from build123d import *

# Parameters (mm, degrees)
SKETCH_1_W      = 44.72
SKETCH_1_H      = 61.65
EXTRUDE_1_DEPTH = 1.125
FILLET_1_R      = 1
SKETCH_2_W      = 37.22
SKETCH_2_H      = 49.65
EXTRUDE_2_DEPTH = 0.78


with BuildPart() as part:
    # 草图1 → 凸台-拉伸1 (new body)
    with BuildSketch(Plane(origin=(0, 0, 0), x_dir=(1, 0, 0), z_dir=(0, 1, 0))):
        with Locations((-1.696923077, -14.271057692)):
            Rectangle(SKETCH_1_W, SKETCH_1_H)
    extrude(amount=EXTRUDE_1_DEPTH)

    # 圆角1
    fillet_1_edges = [part.edges().sort_by_distance(p)[0] for p in [
        (-24.056923077, 0.5625, -16.553942308),
        (20.663076923, 0.5625, -16.553942308),
        (20.663076923, 0.5625, 45.096057692),
        (-24.056923077, 0.5625, 45.096057692),
    ]]
    fillet(fillet_1_edges, radius=FILLET_1_R)

    # 草图2 → 凸台-拉伸2 (add)
    with BuildSketch(Plane.XZ):
        with Locations((-1.696923077, 14.731057692)):
            Rectangle(SKETCH_2_W, SKETCH_2_H)
    extrude(amount=EXTRUDE_2_DEPTH)


solid = part.part
Here's how the part is built. I have some questions about the finished solid (model axes, mm). Coordinates: 2 decimals unless noted, no trailing zeros. Order: outer loops, then holes, each group sorted by start corner. A loop starts at its lowest first (then second) coordinate and runs counter-clockwise, first axis right, second up.
Item 1: If we section it at B-B on x = -5: List the corners of the cut face in (y, z) for me (3 decimals).
Result sheet:
outline: (-0.78, -10.094) - (0, -10.094) - (0, -16.554) - (1.125, -16.554) - (1.125, 45.096) - (0, 45.096) - (0, 39.556) - (-0.78, 39.556) - close
Item 2: If we section it at A-A on z = 25.5: List the corners of the cut face in (x, y) for me (3 decimals).
Result sheet:
outline: (-24.057, 0) - (-20.307, 0) - (-20.307, -0.78) - (16.913, -0.78) - (16.913, 0) - (20.663, 0) - (20.663, 1.125) - (-24.057, 1.125) - close
Item 3: For P1, Ø0.6, axis at x = -5, y = -0.5, coming from the +Z side, with a flat end and sliding along its axis, tell me the tip position at first contact or that it passes through.
Result sheet:
P1: stops at z = 39.56
Item 4: I need wall thicknesses on line 1 (Z direction, x = -4, y = -0.5); line 2 (X direction, y = -0.25, z = 17); line 3 (Y direction, x = 7.5, z = -13.5) (3 decimals). Which ranges of each line are inside material? Lowest first, please.
Result sheet:
line 1: z = -10.09 to 39.56
line 2: x = -20.31 to 16.91
line 3: y = 0 to 1.125
